Print and shaded views of the part. All mm, measured from the part's lowest x, y and z. Round coordinates to 2 decimals unless told otherwise and drop trailing zeros. Loops run counter-clockwise (first coordinate to the right, second up) from the corner with the lowest first, then second, coordinate; pieces in that order, holes last. Notation, with made-up numbers: (-22, 7) - (37, 7) arc R23 cw to (37, 27) - close; hole circle Ø2 at (78, 54). An arc over 180 degrees is marked (long way). Put each result on its own line as item: value. Start each with the question number.
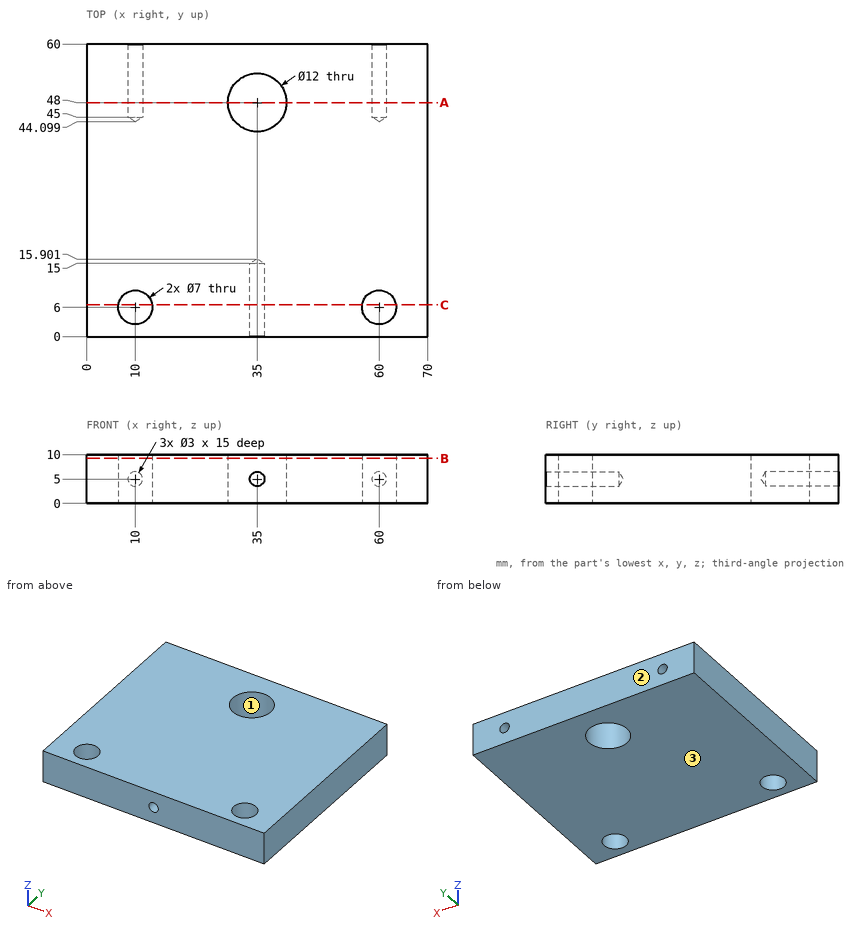
Item 1: Drill centre lines: probe 1 along X at (y, z) = (48, 3.25); probe 2 along Z at (x, y) = (10, 55.5); probe 3 along X at (y, z) = (48, 4.5) (1 decimal). Where is each one in solid material? Low to high. Write a range as [from, to].
Item 2: Slice it at B-B (z = 9.25). Give the cut face in (x, y), plus the area to 3 significant figures.
Item 3: Slice it at C-C (y = 6.5). Give the cut face in (x, z).
Item 4: Two-plate mould, pull along Y, no slides. Class the marked faces 1, 2 and 3: pulls with the +Y half, pulls with the -Y half, needs draft (parallel to the pull), parting line crosses it, or undercut.
Item 5: Drop flat-ended pins along their axis: pin 1 Ø5 at (x, z) = (10, 5) entering from -Y; pin 2 Ø5.5 at (x, y) = (10, 6) entering from +Z; pin 3 Ø2.5 at (x, z) = (60, 5) entering from +Y; pin 4 Ø1.8 at (x, z) = (35, 5) entering from -Y. Give the stop position or say it passes through.
Item 6: Slice it at A-A (y = 48). Give the cut face in (x, z), plus the area to 3 significant figures.
Computed values:
1. probe 1: x = [0, 29], [41, 70]
1. probe 2: z = [0, 3.5], [6.5, 10]
1. probe 3: x = [0, 8.6], [11.4, 29], [41, 58.6], [61.4, 70]
2. outline: (0, 0) - (70, 0) - (70, 60) - (0, 60) - close; hole circle Ø7 at (10, 6); hole circle Ø12 at (35, 48); hole circle Ø7 at (60, 6)
2. area: 4,010 mm^2
3. outline: (0, 0) - (6.54, 0) - (6.54, 10) - (0, 10) - close; (13.46, 0) - (56.54, 0) - (56.54, 10) - (13.46, 10) - close; (63.46, 0) - (70, 0) - (70, 10) - (63.46, 10) - close; hole circle Ø3 at (35, 5)
4. face 1: undercut
4. face 2: pulls with the +Y half
4. face 3: needs draft
5. pin 1: stops at y = 0
5. pin 2: passes through
5. pin 3: stops at y = 44.85
5. pin 4: stops at y = 15.36
6. outline: (0, 0) - (29, 0) - (29, 10) - (0, 10) - close; (41, 0) - (70, 0) - (70, 10) - (41, 10) - close; hole circle Ø3 at (10, 5); hole circle Ø3 at (60, 5)
6. area: 566 mm^2
